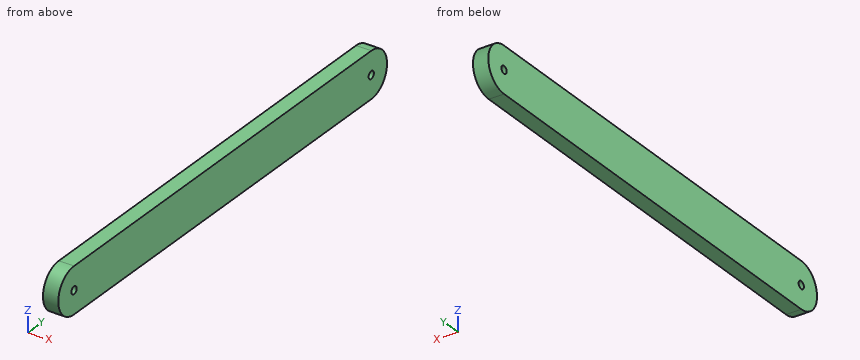
```python
from build123d import *

# Parameters (mm, degrees)
EXTRUDE_1_DEPTH     = 10
SKETCH_3_R          = 2.5
CUT_EXTRUDE_1_DEPTH = 10


with BuildPart() as part:
    # 草图2 → 凸台-拉伸1 (new body)
    with BuildSketch(Plane(origin=(0, 0, 0), x_dir=(0, 0, -1), z_dir=(1, 0, 0))):
        with BuildLine():
            Line((0, 0), (0, 282.909))
            ThreePointArc((0, 282.909), (15, 297.909), (30, 282.909))
            Line((30, 282.909), (30, 0))
            ThreePointArc((30, 0), (15, -15), (0, 0))
        make_face()
    extrude(amount=EXTRUDE_1_DEPTH)

    # 草图3 → 切除-拉伸1 (cut)
    with BuildSketch(Plane.ZY):
        with Locations((-15, 0)):
            Circle(SKETCH_3_R)
        with Locations(Location((-15, 282.909, 0), (0, 0, 180))):
            Circle(SKETCH_3_R)
    extrude(amount=-CUT_EXTRUDE_1_DEPTH, mode=Mode.SUBTRACT)


solid = part.part
```
Geometry: final body of the model. Coordinates: model frame, mm. Give positions to 0.01 mm unless a question says otherwise; leave off trailing zeros. Loops run counter-clockwise (first coordinate to the right, second up) from the corner with the lowest first, then second, coordinate; pieces in that order, holes last. Notation, with made-up numbers: (47.5, -38.5) - (63.5, -38.5) arc R23 ccw to (63.5, -18.5) - close; hole circle Ø7 at (58.5, 55.25). An arc over 180 degrees is marked (long way). Answer as CSV lines item,"result". Start each with the question number.
(1) Section query B-B (z = -4.25). Output: boundary loops of the cut face in (x, y), and give its area (3 significant figures).
(2) Section query A-A (x = 6.75). Output: boundary loops of the cut face in (y, z), and give its area (3 significant figures).
(3) Pin query (flat end, axial travel): P1, Ø4, axis at y = 0, z = -15, coming from the +X side; P2, Ø6, axis at y = 263, z = -11, coming from the -X side; P3, Ø5, axis at x = 1.5, z = -5, coming from the +Y side; P4, Ø4, axis at x = 1.5, z = -24, coming from the -Y side. Return the tip coordinate at first contact, or that it passes through.
(4) Ray query, line 1 along Y through (x, z) = (5, -15); line 2 along Y through (x, z) = (6.5, -14.5); line 3 along Z through (x, y) = (0.75, 281). Return the intervals inside material, ascending. Write a range as [from, to].
Worked answers:
1,outline,"(0, -10.46) - (10, -10.46) - (10, 293.37) - (0, 293.37) - close"
1,area,"3,040 mm^2"
2,outline,"(0, -30) - (282.91, -30) arc R15 ccw to (282.91, 0) - (0, 0) arc R15 ccw to start; hole circle Ø5 at (0, -15); hole circle Ø5 at (282.91, -15)"
2,area,"9,150 mm^2"
3,P1,"passes through"
3,P2,"stops at x = 0"
3,P3,"stops at y = 295.9"
3,P4,"stops at y = -13.27"
4,line 1,"y = [-15, -2.5], [2.5, 280.41], [285.41, 297.91]"
4,line 2,"y = [-14.99, -2.45], [2.45, 280.46], [285.36, 297.9]"
4,line 3,"z = [-30, -16.61], [-13.39, 0]"
